```python
from build123d import *

# Parameters (mm, degrees)
BOSS_EXTRUDE4_DEPTH = 5
SKETCH6_W           = 70
SKETCH6_H           = 70
BOSS_EXTRUDE5_DEPTH = 30
SKETCH8_R           = 3
CUT_EXTRUDE1_DEPTH  = 2
FILLET1_R           = 7.5
CUT_EXTRUDE2_DEPTH  = 27.5
CHAMFER1_SIZE       = 1.25
CHAMFER2_SIZE       = 1.25


with BuildPart() as part:
    # Sketch5 → Boss-Extrude4 (new body)
    with BuildSketch(Plane(origin=(0, 0, 0), x_dir=(1, 0, 0), z_dir=(0, 1, 0))):
        with BuildLine():
            Line((-22.5, -32.5), (22.5, -32.5))
            ThreePointArc((22.5, -32.5), (29.571067812, -29.571067812), (32.5, -22.5))
            Line((32.5, -22.5), (32.5, 22.5))
            ThreePointArc((32.5, 22.5), (29.571067812, 29.571067812), (22.5, 32.5))
            Line((22.5, 32.5), (-22.5, 32.5))
            ThreePointArc((-22.5, 32.5), (-29.571067812, 29.571067812), (-32.5, 22.5))
            Line((-32.5, 22.5), (-32.5, -22.5))
            ThreePointArc((-32.5, -22.5), (-29.571067812, -29.571067812), (-22.5, -32.5))
        make_face()
    extrude(amount=BOSS_EXTRUDE4_DEPTH)

    # Sketch6 → Boss-Extrude5 (add)
    with BuildSketch(Plane(origin=(0, 5, 0), x_dir=(1, 0, 0), z_dir=(0, 1, 0))):
        Rectangle(SKETCH6_W, SKETCH6_H)
    extrude(amount=BOSS_EXTRUDE5_DEPTH)

    # Sketch8 → Cut-Extrude1 (cut)
    with BuildSketch(Plane.XZ):
        with Locations(Location((26.037533906, -26.035533906, 0), (0, 0, 270))):
            Circle(SKETCH8_R)
        with Locations(Location((26.036533906, 26.036533906, 0), (0, 0, 270))):
            Circle(SKETCH8_R)
        with BuildLine():
            ThreePointArc((-23.035533906, 26.035533906), (-24.887483609, 28.807172503), (-28.156854249, 28.156854249))
            Line((-28.156854249, 28.156854249), (-23.914213562, 23.914213562))
            ThreePointArc((-23.914213562, 23.914213562), (-23.263895308, 24.887483609), (-23.035533906, 26.035533906))
        make_face()
        with BuildLine():
            Line((-23.914213562, 23.914213562), (-28.156854249, 28.156854249))
            ThreePointArc((-28.156854249, 28.156854249), (-28.156854249, 23.914213562), (-23.914213562, 23.914213562))
        make_face()
        with Locations(Location((-26.034533906, -26.036533906, 0), (0, 0, 270))):
            Circle(SKETCH8_R)
    extrude(amount=-CUT_EXTRUDE1_DEPTH, mode=Mode.SUBTRACT)

    # Mirror1: part across plane


with BuildPart() as part_1:
    add(part.part)
    add(part.part.mirror(Plane(origin=(-35, 35, -35), x_dir=(0, 0, 1), z_dir=(1, 0, 0))))

    # Mirror2: part across plane


with BuildPart() as part_2:
    add(part_1.part)
    add(part_1.part.mirror(Plane(origin=(35, 35, 35), x_dir=(1, 0, 0), z_dir=(0, 0, -1))))

    # Fillet1
    fillet1_edges = [part_2.edges().sort_by_distance(p)[0] for p in [
        (35, 20, 105),
        (-105, 20, 105),
        (35, 20, -35),
        (-105, 20, -35),
    ]]
    fillet(fillet1_edges, radius=FILLET1_R)

    # Sketch11 → Cut-Extrude2 (cut)
    with BuildSketch(Plane(origin=(0, 35, 0), x_dir=(1, 0, 0), z_dir=(0, 1, 0))):
        with BuildLine():
            Line((32.5, -97.5), (32.5, 27.5))
            ThreePointArc((32.5, 27.5), (31.035533906, 31.035533906), (27.5, 32.5))
            Line((27.5, 32.5), (-97.5, 32.5))
            ThreePointArc((-97.5, 32.5), (-101.035533906, 31.035533906), (-102.5, 27.5))
            Line((-102.5, 27.5), (-102.5, -97.5))
            ThreePointArc((-102.5, -97.5), (-101.035533906, -101.035533906), (-97.5, -102.5))
            Line((-97.5, -102.5), (27.5, -102.5))
            ThreePointArc((27.5, -102.5), (31.035533906, -101.035533906), (32.5, -97.5))
        make_face()
    extrude(amount=-CUT_EXTRUDE2_DEPTH, mode=Mode.SUBTRACT)

    # Chamfer1
    chamfer1_edges = [part_2.edges().sort_by_distance(p)[0] for p in [
        (31.035533906, 7.5, -31.035533906),
        (32.5, 7.5, 35),
        (31.035533906, 7.5, 101.035533906),
        (-35, 7.5, 102.5),
        (-101.035533906, 7.5, 101.035533906),
        (-102.5, 7.5, 35),
        (-101.035533906, 7.5, -31.035533906),
        (-35, 7.5, -32.5),
        (31.035533906, 35, -31.035533906),
        (-35, 35, -32.5),
        (-101.035533906, 35, -31.035533906),
        (-102.5, 35, 35),
        (-101.035533906, 35, 101.035533906),
        (-35, 35, 102.5),
        (31.035533906, 35, 101.035533906),
        (32.5, 35, 35),
    ]]
    chamfer(chamfer1_edges, length=CHAMFER1_SIZE)

    # Chamfer2
    chamfer2_edges = [part_2.edges().sort_by_distance(p)[0] for p in [
        (32.5, 0, 0),
        (29.571067812, 0, 29.571067812),
        (0, 0, 32.5),
        (-29.571067812, 0, 29.571067812),
        (-29.571067812, 0, 40.428932188),
        (0, 0, 37.5),
        (29.571067812, 0, 40.428932188),
        (32.5, 0, 70),
        (29.571067812, 0, 99.571067812),
        (0, 0, 102.5),
        (-29.571067812, 0, 99.571067812),
        (-32.5, 0, 70),
        (-40.428932188, 0, 40.428932188),
        (-70, 0, 37.5),
        (-99.571067812, 0, 40.428932188),
        (-102.5, 0, 70),
        (-99.571067812, 0, 99.571067812),
        (-70, 0, 102.5),
        (-40.428932188, 0, 99.571067812),
        (-37.5, 0, 70),
        (-35, 5, -35),
        (35, 5, 35),
        (-35, 5, 105),
        (-105, 5, 35),
        (-102.803300859, 5, 102.803300859),
        (-102.803300859, 5, -32.803300859),
        (32.803300859, 5, 102.803300859),
        (32.803300859, 5, -32.803300859),
        (-40.428932188, 0, 29.571067812),
        (-70, 0, 32.5),
        (-99.571067812, 0, 29.571067812),
        (-102.5, 0, 0),
        (-99.571067812, 0, -29.571067812),
        (-70, 0, -32.5),
        (-40.428932188, 0, -29.571067812),
        (-37.5, 0, 0),
        (-32.5, 0, 0),
        (-29.571067812, 0, -29.571067812),
        (0, 0, -32.5),
        (29.571067812, 0, -29.571067812),
    ]]
    chamfer(chamfer2_edges, length=CHAMFER2_SIZE)


solid = part_2.part
```
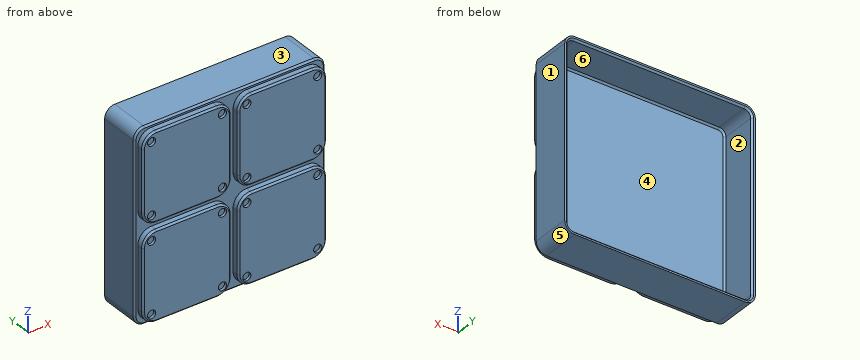
For this review, take the finished solid that the model builds, in its own axes (mm). Face numbers are marked on the shaded views. A direction names the side the tool comes from. Round coordinates to 2 decimals unless told otherwise and drop trailing zeros. Order: outer loops, then holes, each group sorted by start corner. A loop starts at its lowest first (then second) coordinate and runs counter-clockwise, first axis right, second up.
Q1. We need section C-C, the plane z = 66.5. Give the boundary of the cut face in (x, y), plus the area to 3 significant figures.
Findings below:
outline: (-105, 6.25) - (-103.75, 5) - (-102.5, 5) - (-102.5, 1.25) - (-101.25, 0) - (-38.75, 0) - (-37.5, 1.25) - (-37.5, 5) - (-32.5, 5) - (-32.5, 1.25) - (-31.25, 0) - (31.25, 0) - (32.5, 1.25) - (32.5, 5) - (33.75, 5) - (35, 6.25) - (35, 35) - (33.75, 35) - (32.5, 33.75) - (32.5, 8.75) - (31.25, 7.5) - (-101.25, 7.5) - (-102.5, 8.75) - (-102.5, 33.75) - (-103.75, 35) - (-105, 35) - close
area: 1,130 mm2
Q2. Insertion check: P1, Ø1.5, axis at x = -64.5, z = -18, coming from the +Y side; P2, Ø3, axis at x = -25, z = 96, coming from the -Y side; P3, Ø1.1, axis at x = -1, y = 2.5, coming from the -Z side. Each pin has a flat end and moves straight along its axis. Give the tip position at first contact, or say it passes through.
Findings below:
P1: stops at y = 7.5
P2: stops at y = 2
P3: stops at z = -32.5
Q3. Wall thickness on line 1 (X direction, y = 12, z = 88); line 2 (Z direction, x = -39, y = 16.5); line 3 (Z direction, x = -47.5, y = 2.5): over which ranges is each line inside the solid? List them lowest first.
Findings below:
line 1: x = -105 to -102.5, 32.5 to 35
line 2: z = -35 to -32.5, 102.5 to 105
line 3: z = -32.5 to 32.5, 37.5 to 102.5
Q4. Mouldability with a two-part tool opening along X and no side actions: class the marked faces 3, 4, 5 and 6 as pulls with the +X half, pulls with the -X half, needs draft (parallel to the pull), parting line crosses it, or undercut.
Findings below:
face 3: needs draft
face 4: undercut
face 5: pulls with the +X half
face 6: undercut
Q5. Machinability: for the marked faces 1 and 2, which of the approach directions +Z, -Z, +X, -X, +Y, -Y give a long, thin tool a straight path to every point of the face, cutting with its end or side? Answer none if there is none.
Findings below:
face 1: +Z, -Z, +X, +Y, -Y
face 2: +Y
Q6. We need section A-A, the plane y = 11.5. Give the boundary of the cut face in (x, z).
Findings below:
outline: (-105, -27.5) arc R7.5 ccw to (-97.5, -35) - (27.5, -35) arc R7.5 ccw to (35, -27.5) - (35, 97.5) arc R7.5 ccw to (27.5, 105) - (-97.5, 105) arc R7.5 ccw to (-105, 97.5) - close; hole (-102.5, -27.5) arc R5 ccw to (-97.5, -32.5) - (27.5, -32.5) arc R5 ccw to (32.5, -27.5) - (32.5, 97.5) arc R5 ccw to (27.5, 102.5) - (-97.5, 102.5) arc R5 ccw to (-102.5, 97.5) - close
Q7. We need section B-B, the plane x = 6.5. Give the boundary of the cut face in (y, z).
Findings below:
outline: (0, -31.25) - (1.25, -32.5) - (5, -32.5) - (5, -33.75) - (6.25, -35) - (35, -35) - (35, -33.75) - (33.75, -32.5) - (8.75, -32.5) - (7.5, -31.25) - (7.5, 101.25) - (8.75, 102.5) - (33.75, 102.5) - (35, 103.75) - (35, 105) - (6.25, 105) - (5, 103.75) - (5, 102.5) - (1.25, 102.5) - (0, 101.25) - (0, 38.75) - (1.25, 37.5) - (5, 37.5) - (5, 32.5) - (1.25, 32.5) - (0, 31.25) - close
